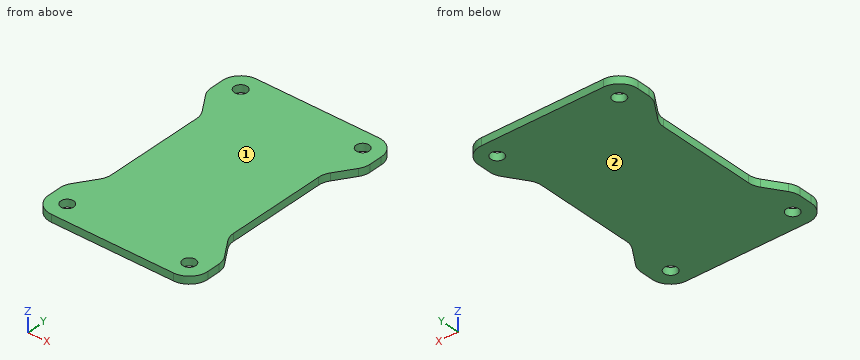
from build123d import *

# Parameters (mm, degrees)
F1_DEPTH = 2
F2_R     = 1.75
F3_DEPTH = 25
F4_R     = 5


with BuildPart() as f1:
    # F0 (on Top) → F1 (new body)
    with BuildSketch(Plane.XY):
        Polygon((21.5, 32.5), (-21.5, 32.5), (-21.5, 22.5), (-16.5, 15), (-16.5, -15), (-21.5, -22.5), (-21.5, -32.5), (21.5, -32.5), (21.5, -22.5), (16.5, -15), (16.5, 15), (21.5, 22.5), align=None)
    extrude(amount=F1_DEPTH)

    # F2 (on Top) → F3 (cut)
    with BuildSketch(Plane.XY):
        with Locations((-16.5, 27.5)):
            Circle(F2_R)
        with Locations((16.5, 27.5)):
            Circle(F2_R)
        with Locations((16.5, -27.5)):
            Circle(F2_R)
        with Locations((-16.5, -27.5)):
            Circle(F2_R)
    extrude(amount=F3_DEPTH, mode=Mode.SUBTRACT)

    # F4
    f4_edges = [f1.edges().sort_by_distance(p)[0] for p in [
        (-21.5, 32.5, 1),
        (21.5, 32.5, 1),
        (21.5, -32.5, 1),
        (-21.5, -32.5, 1),
        (21.5, 22.5, 1),
        (16.5, 15, 1),
        (16.5, -15, 1),
        (21.5, -22.5, 1),
        (-21.5, -22.5, 1),
        (-16.5, -15, 1),
        (-16.5, 15, 1),
        (-21.5, 22.5, 1),
    ]]
    fillet(f4_edges, radius=F4_R)


solid = f1.part
Could you check a few things on this model? Use its own coordinates, in mm. Face numbers are marked on the shaded views. Give positions to 0.01 mm unless a question says otherwise; leave off trailing zeros. Write each loop counter-clockwise with the first axis right and the second up, starting at its lowest first coordinate (ties: lowest second). Pieces come first, ordered by that corner, then holes. Notation, with made-up numbers: (-38, 4) -> (-19, 4) arc R35 cw to (-19, 38) -> close; hole circle Ø3 at (-16.5, 54.5). An arc over 180 degrees is marked (long way). Answer as CSV lines item,"result". Start each with the question number.
(1) If we section it at C-C, the plane y = 4.5: Write out the boundary of the cut face in (x, z).
(2) If we section it at A-A, the plane z = 1.65: Write out the boundary of the cut face in (x, y), and give its area (3 significant figures).
(3) If we mould it in two halves opening along Z, with no side actions, what happens to the marked faces 1 and 2? For each: +Z half, -Z half, draft (parallel to the pull), parting line (faces both ways), or undercut.
(4) Please list where these lines run through material, in increasing order: line 1 (X direction, y = 27.5, z = 1.5); line 2 (X direction, y = 26, z = 0.55); line 3 (X direction, y = 5, z = 0.4).
(5) If we section it at B-B, the plane x = 15.5: Write out the boundary of the cut face in (y, z), and give its area (3 significant figures).
(6) I'm going to push flat-ended pins straight in: pin 1 Ø1 at (y, z) = (3.5, 1.5) entering from +X; pin 2 Ø3 at (x, y) = (16.5, 27.5) entering from +Z; pin 3 Ø4 at (x, y) = (-16.5, -27.5) entering from -Z. Where does each tip first touch, or does it pass through?
Answer list:
1,outline,"(-16.5, 0) -> (16.5, 0) -> (16.5, 2) -> (-16.5, 2) -> close"
2,outline,"(-21.5, -27.5) arc R5 ccw to (-16.5, -32.5) -> (16.5, -32.5) arc R5 ccw to (21.5, -27.5) -> (21.5, -24.01) arc R5 ccw to (20.66, -21.24) -> (17.34, -16.26) arc R5 cw to (16.5, -13.49) -> (16.5, 13.49) arc R5 cw to (17.34, 16.26) -> (20.66, 21.24) arc R5 ccw to (21.5, 24.01) -> (21.5, 27.5) arc R5 ccw to (16.5, 32.5) -> (-16.5, 32.5) arc R5 ccw to (-21.5, 27.5) -> (-21.5, 24.01) arc R5 ccw to (-20.66, 21.24) -> (-17.34, 16.26) arc R5 cw to (-16.5, 13.49) -> (-16.5, -13.49) arc R5 cw to (-17.34, -16.26) -> (-20.66, -21.24) arc R5 ccw to (-21.5, -24.01) -> close; hole circle Ø3.5 at (-16.5, -27.5); hole circle Ø3.5 at (-16.5, 27.5); hole circle Ø3.5 at (16.5, -27.5); hole circle Ø3.5 at (16.5, 27.5)"
2,area,"2,360 mm^2"
3,face 1,"+Z half"
3,face 2,"-Z half"
4,line 1,"-21.5 to -18.25, -14.75 to 14.75, 18.25 to 21.5"
4,line 2,"-21.5 to -17.4, -15.6 to 15.6, 17.4 to 21.5"
4,line 3,"-16.5 to 16.5"
5,outline,"(-32.5, 0) -> (-28.94, 0) -> (-28.94, 2) -> (-32.5, 2) -> close; (-26.06, 0) -> (26.06, 0) -> (26.06, 2) -> (-26.06, 2) -> close; (28.94, 0) -> (32.5, 0) -> (32.5, 2) -> (28.94, 2) -> close"
5,area,"119 mm^2"
6,pin 1,"x = 16.5"
6,pin 2,"through"
6,pin 3,"z = 0"
